from build123d import *

# Parameters (mm, degrees)
CROQUIS1_W              = 12
CROQUIS1_H              = 10
SALIENTE_EXTRUIR1_DEPTH = 20
CHAFL_N1_SIZE           = 0.5


with BuildPart() as part:
    # Croquis1 → Saliente-Extruir1 (new body, symmetric)
    with BuildSketch(Plane.XY):
        Rectangle(CROQUIS1_W, CROQUIS1_H)
    extrude(amount=SALIENTE_EXTRUIR1_DEPTH, both=True)

    # Croquis3 → Cortar-Revolución1 (revolve, cut)
    with BuildSketch(Plane.XY.offset(-14)):
        Polygon((0, 5), (-2.25, 5), (-2.25, -3.2), (-4, -5), (0, -5), align=None)
    cortar_revoluci_n1 = revolve(axis=Axis((0, 5, -14), (0, -1, 0)), mode=Mode.SUBTRACT)

    # Simetría1: Cortar-Revolución1 across plane
    add(cortar_revoluci_n1.mirror(Plane.XY), mode=Mode.SUBTRACT)

    # Chaflán1
    chafl_n1_edges = [part.edges().sort_by_distance(p)[0] for p in [
        (6, 0, 20),
        (0, 5, 20),
        (-6, 0, 20),
        (0, 5, -20),
        (6, 0, -20),
        (0, -5, -20),
        (-6, 0, -20),
        (0, -5, 20),
        (-6, 5, 0),
        (6, 5, 0),
        (6, -5, 0),
        (-6, -5, 0),
    ]]
    chamfer(chafl_n1_edges, length=CHAFL_N1_SIZE)


solid = part.part
Read the model definition and answer for the solid it produces. Units are mm, in the model's axes. Coordinates: 2 decimals unless noted, no trailing zeros. Order: outer loops, then holes, each group sorted by start corner. A loop starts at its lowest first (then second) coordinate and runs counter-clockwise, first axis right, second up. Notation, with made-up numbers: (-24.75, -15) -> (24.25, -15) arc R24 ccw to (24.25, -1) -> close; hole circle Ø4 at (-28, -29.75). An arc over 180 degrees is marked (long way). Answer as a JSON object with one key per item and string values.
1) This flat-tipped pin is pushed along its axis until it touches: pin 1 (6 mm diameter, centred on x = 0, z = -14, fed in from +Y). Where does it stop, or does it pass through?
Model answer:
{"pin 1": "stops at y = 5"}
2) The mould has two halves that part along Z. Classify faces 1 (the face through (0.488, 0.843, 11.804)), 2 (the face through (-6, 0, 0)), 3 (the face through (0, 0, -20)), 4 (the face through (0.488, 0.843, -11.804)): released by +Z, released by -Z, zero draft, split by the parting line, or undercut.
Model answer:
{"face 1": "undercut", "face 2": "zero draft", "face 3": "released by -Z", "face 4": "undercut"}
3) Consider line 1 along Z through (x, y) = (0, 1.75); line 2 along X through (y, z) = (0, -14); line 3 along Z through (x, y) = (-2, -3). Determine where each line is inside the solid, lowest interval first. Write a range as from..to.
Model answer:
{"line 1": "z = -20..-16.25, -11.75..11.75, 16.25..20", "line 2": "x = -6..-2.25, 2.25..6", "line 3": "z = -20..-15.03, -12.97..12.97, 15.03..20"}
4) A cutting plane is placed at C-C, the plane x = 0. Determine the outline of the cut face in (y, z).
Model answer:
{"outline": "(-5, -19.5) -> (-4.5, -20) -> (4.5, -20) -> (5, -19.5) -> (5, -16.25) -> (-3.2, -16.25) -> (-5, -18) -> close; (-5, -10) -> (-3.2, -11.75) -> (5, -11.75) -> (5, 11.75) -> (-3.2, 11.75) -> (-5, 10) -> close; (-5, 18) -> (-3.2, 16.25) -> (5, 16.25) -> (5, 19.5) -> (4.5, 20) -> (-4.5, 20) -> (-5, 19.5) -> close"}
5) A cutting plane is placed at B-B, the plane y = 2. Determine the outline of the cut face in (x, z), plus the area to 3 significant figures.
Model answer:
{"outline": "(-6, -19.5) -> (-5.5, -20) -> (5.5, -20) -> (6, -19.5) -> (6, 19.5) -> (5.5, 20) -> (-5.5, 20) -> (-6, 19.5) -> close; hole circle Ø4.5 at (0, -14); hole circle Ø4.5 at (0, 14)", "area": "448 mm²"}
6) A cutting plane is placed at A-A, the plane z = 14. Determine the outline of the cut face in (x, y), plus the area to 4 significant figures.
Model answer:
{"outline": "(-6, -4.5) -> (-5.5, -5) -> (-4, -5) -> (-2.25, -3.2) -> (-2.25, 5) -> (-5.5, 5) -> (-6, 4.5) -> close; (2.25, -3.2) -> (4, -5) -> (5.5, -5) -> (6, -4.5) -> (6, 4.5) -> (5.5, 5) -> (2.25, 5) -> close", "area": "71.35 mm²"}
